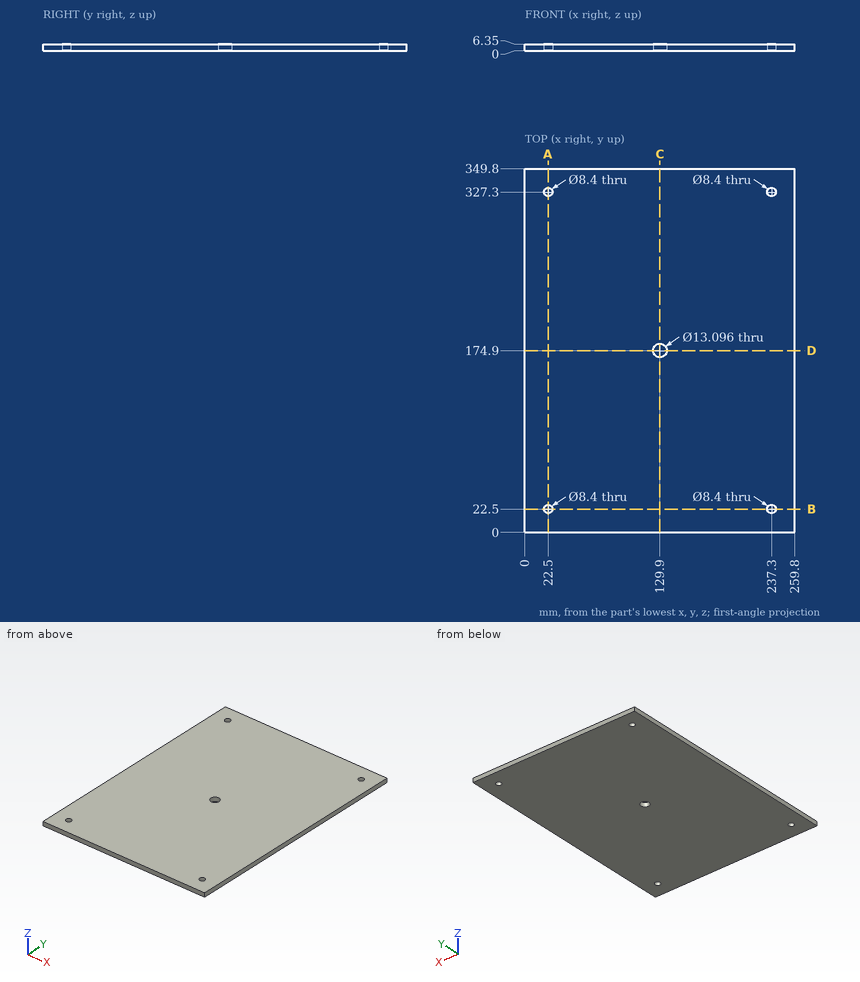
Here's the drawing with two shaded views (mm, measured from the low corner). I have some questions. Round coordinates to 2 decimals unless told otherwise and drop trailing zeros. Loops run counter-clockwise (first coordinate to the right, second up) from the corner with the lowest first, then second, coordinate; pieces in that order, holes last.
1. Suppose I cut it at A-A, the plane x = 22.5. Please give me the cut outline in (y, z).
Answers:
outline: (0, 0) - (18.3, 0) - (18.3, 6.35) - (0, 6.35) - close; (26.7, 0) - (323.1, 0) - (323.1, 6.35) - (26.7, 6.35) - close; (331.5, 0) - (349.8, 0) - (349.8, 6.35) - (331.5, 6.35) - close
2. Suppose I cut it at B-B, the plane y = 22.5. Please give me the cut outline in (x, z), and give its area (3 significant figures).
Answers:
outline: (0, 0) - (18.3, 0) - (18.3, 6.35) - (0, 6.35) - close; (26.7, 0) - (233.1, 0) - (233.1, 6.35) - (26.7, 6.35) - close; (241.5, 0) - (259.8, 0) - (259.8, 6.35) - (241.5, 6.35) - close
area: 1,540 mm2
3. Suppose I cut it at C-C, the plane x = 129.9. Please give me the cut outline in (y, z).
Answers:
outline: (0, 0) - (168.35, 0) - (168.35, 6.35) - (0, 6.35) - close; (181.45, 0) - (349.8, 0) - (349.8, 6.35) - (181.45, 6.35) - close
4. Will these pins go through, and if not, where does the flat tip stop? pin 1 (17 mm diameter, centred on x = 129.9, y = 174.9, fed in from +Z); pin 2 (7.5 mm diameter, centred on x = 237.3, y = 327.3, fed in from -Z).
Answers:
pin 1: stops at z = 6.35
pin 2: passes through
5. If I drill on probe 1 along X at (y, z) = (327.3, 3.5); probe 2 along Y at (x, z) = (237.3, 4); probe 3 along X at (y, z) = (325.5, 6.25) (1 decimal), over which ranges is the centre line in solid material (lowest first)?
Answers:
probe 1: x = 0 to 18.3, 26.7 to 233.1, 241.5 to 259.8
probe 2: y = 0 to 18.3, 26.7 to 323.1, 331.5 to 349.8
probe 3: x = 0 to 18.7, 26.3 to 233.5, 241.1 to 259.8
6. Suppose I cut it at D-D, the plane y = 174.9. Please give me the cut outline in (x, z), and give its area (3 significant figures).
Answers:
outline: (0, 0) - (123.35, 0) - (123.35, 6.35) - (0, 6.35) - close; (136.45, 0) - (259.8, 0) - (259.8, 6.35) - (136.45, 6.35) - close
area: 1,570 mm2
